Geometry: final body of the model. Coordinates: model frame, mm. A direction names the side the tool comes from. Give positions to 0.01 mm unless a question says otherwise; leave off trailing zeros. Write each loop counter-clockwise with the first axis right and the second up, starting at its lowest first coordinate (ties: lowest second). Pieces come first, ordered by that corner, then holes. Notation, with made-up numbers: M 30.25,73.5 L 59.25,73.5 A25 ccw 59.25,109.5 Z; hole C -34.5,-9.5 d11. An arc over 180 degrees is marked long. Use a Markdown table: item, result. Add a question column.
(1) Cut plane C-C (y = -119). Output: boundary loops of the cut face in (x, z), plus the area to 3 significant figures.
(2) Draft query along X for faces 1 (the flat face through (-66, -209.75, 86)), 2 (the cylindrical face through (-156.251, -140.305, 85.782)), 3 (the flat face through (163.933, -96, 86)), 4 (the cylindrical face through (185.99, -96.97, 85.78)). Return one class per face: released by +X, released by -X, zero draft, split by the parting line, or undercut.
(3) Material intervals for L1, parallel to X at y = -180, z = 83.5; L2, parallel to X at y = -142.5, z = 125; L3, parallel to Y at x = -4, z = 110.5, sorted ascending.
(4) Cut plane D-D (x = -28). Output: boundary loops of the cut face in (y, z).
(5) Pin query (flat end, axial travel): pin 1 Ø5 at (x, z) = (-42.5, 114.5) entering from -Y; pin 2 Ø10 at (x, z) = (-94.5, 102) entering from +Y; pin 3 Ø1.2 at (x, z) = (-166.5, 130) entering from -Y. Return the tip coordinate at first contact, or that it passes through.
(6) Cut plane B-B (z = 146.5). Output: boundary loops of the cut face in (x, y), plus the area to 3 significant figures.
(7) Cut plane A-A (y = -168). Output: boundary loops of the cut face in (x, z), plus the area to 3 significant figures.
(8) Reachability of faces 5 (the flat face through (-13, -199, 174)), 6 (the flat face through (120, -191, 86)), 7 (the flat face through (-163.933, -95, 86)), 8 (the flat face through (-120, -191, 86)) from +Z, -Z, +X, -X, +Y, -Y: full face, straight path, thin tool, end or side. Return the list, or none.
```python
from build123d import *

# Parameters (mm, degrees)
SKETCH_1_R          = 210
SKETCH_1_R_2        = 203
EXTRUDE_2_DEPTH     = 174
EXTRUDE_START       = -174
EXTRUDE_4_DEPTH     = 174
CUT_EXTRUDE_1_DEPTH = 654
EXTRUDE_5_DEPTH     = 174
EXTRUDE_6_DEPTH     = 174
EXTRUDE_7_DEPTH     = 174
EXTRUDE_8_DEPTH     = 174


with BuildPart() as part:
    # 草图1 → 凸台-拉伸2 (new body)
    with BuildSketch(Plane.XY):
        Circle(SKETCH_1_R)
        Circle(SKETCH_1_R_2, mode=Mode.SUBTRACT)
    extrude(amount=EXTRUDE_2_DEPTH)

    # 草图2 → 凸台-拉伸4 (add)
    with BuildSketch(Plane.XY.offset(174).offset(EXTRUDE_START)):
        with BuildLine():
            Line((-170.735431044, -102), (-173.735431044, -102))
            Line((-173.735431044, -102), (-175.513532242, -102))
            ThreePointArc((-175.513532242, -102), (-174.63092392, -103.50381834), (-173.735431044, -105))
            Line((-173.735431044, -105), (-170.735431044, -105))
            Line((-170.735431044, -105), (-170.735431044, -102))
        make_face()
        with BuildLine():
            ThreePointArc((173.735431044, -105), (174.63092392, -103.50381834), (175.513532242, -102))
            Line((175.513532242, -102), (173.735431044, -102))
            Line((173.735431044, -102), (170.735431044, -102))
            Line((170.735431044, -102), (170.735431044, -105))
            Line((170.735431044, -105), (173.735431044, -105))
        make_face()
    extrude(amount=EXTRUDE_4_DEPTH)

    # 草图3 → 切除-拉伸1 (cut)
    with BuildSketch(Plane.XY.offset(174)):
        Polygon((-170.735431044, -102), (238.333646515, -102), (254.334169784, 272.292523591), (-334.569415043, 221.85110305), (-306.830562533, -102), align=None)
    extrude(amount=-CUT_EXTRUDE_1_DEPTH, mode=Mode.SUBTRACT)

    # 草图5 → 凸台-拉伸5 (add)
    with BuildSketch(Plane.XY.offset(174).offset(EXTRUDE_START)):
        with BuildLine():
            Line((-120, -209.75), (-10.243900624, -209.75))
            ThreePointArc((-10.243900624, -209.75), (-67.755470707, -198.769203322), (-120, -172.336879396))
            Line((-120, -172.336879396), (-120, -209.75))
        make_face()
        with BuildLine():
            ThreePointArc((120, -172.336879396), (67.755470707, -198.769203322), (10.243900624, -209.75))
            Line((10.243900624, -209.75), (120, -209.75))
            Line((120, -209.75), (120, -172.336879396))
        make_face()
    extrude(amount=EXTRUDE_5_DEPTH)

    # 草图6 → 凸台-拉伸6 (add)
    with BuildSketch(Plane.XY.offset(174).offset(EXTRUDE_START)):
        with BuildLine():
            Line((-175.513532242, -102), (-166.195667814, -102))
            ThreePointArc((-166.195667814, -102), (0, -195), (166.195667814, -102))
            Line((166.195667814, -102), (175.513532242, -102))
            ThreePointArc((175.513532242, -102), (0, -203), (-175.513532242, -102))
        make_face()
    extrude(amount=EXTRUDE_6_DEPTH)

    # 草图7 → 凸台-拉伸7 (add)
    with BuildSketch(Plane.XY.offset(174).offset(EXTRUDE_START)):
        with BuildLine():
            Line((-166.933126535, -92), (-166.933126535, -95))
            Line((-166.933126535, -95), (-170.293863659, -95))
            ThreePointArc((-170.293863659, -95), (0, -195), (170.293863659, -95))
            Line((170.293863659, -95), (166.933126535, -95))
            Line((166.933126535, -95), (166.933126535, -92))
            Line((166.933126535, -92), (171.933126535, -92))
            Line((171.933126535, -92), (188.496850106, -92))
            ThreePointArc((188.496850106, -92), (0, -209.75), (-188.496850106, -92))
            Line((-188.496850106, -92), (-171.933126535, -92))
            Line((-171.933126535, -92), (-166.933126535, -92))
        make_face()
    extrude(amount=EXTRUDE_7_DEPTH)

    # 草图8 → 凸台-拉伸8 (add)
    with BuildSketch(Plane(origin=(0, 0, 0), x_dir=(-1, 0, 0), z_dir=(0, 0, -1))):
        with BuildLine():
            Line((166.933126535, -92), (163.933126535, -92))
            Line((163.933126535, -92), (163.933126535, -99))
            Line((163.933126535, -99), (168, -99))
            ThreePointArc((168, -99), (169.158755456, -97.006780447), (170.293863659, -95))
            Line((170.293863659, -95), (166.933126535, -95))
            Line((166.933126535, -95), (166.933126535, -92))
        make_face()
        with BuildLine():
            Line((-166.933126535, -95), (-170.293863659, -95))
            ThreePointArc((-170.293863659, -95), (-169.158755456, -97.006780447), (-168, -99))
            Line((-168, -99), (-163.933126535, -99))
            Line((-163.933126535, -99), (-163.933126535, -92))
            Line((-163.933126535, -92), (-166.933126535, -92))
            Line((-166.933126535, -92), (-166.933126535, -95))
        make_face()
    extrude(amount=-EXTRUDE_8_DEPTH)


solid = part.part
```
Answer list:
| question | item | result |
|---|---|---|
| 1 | outline | M -173.03,0 L -154.48,0 L -154.48,174 L -173.03,174 Z; M 154.48,0 L 173.03,0 L 173.03,174 L 154.48,174 Z |
| 1 | area | 6,460 mm² |
| 2 | face 1 | zero draft |
| 2 | face 2 | released by -X |
| 2 | face 3 | undercut |
| 2 | face 4 | released by +X |
| 3 | L1 | -120 to -75, 75 to 120 |
| 3 | L2 | -154.25 to -133.11, 133.11 to 154.25 |
| 3 | L3 | -209.96 to -194.96 |
| 4 | outline | M -209.75,0 L -192.98,0 L -192.98,174 L -209.75,174 Z |
| 5 | pin 1 | y = -209.75 |
| 5 | pin 2 | y = -167.7 |
| 5 | pin 3 | y = -128.75 |
| 6 | outline | M -188.5,-92 A209.75 ccw -183.28,-102 L -183.56,-102 A210 ccw -120,-172.34 L -120,-209.75 L -10.24,-209.75 A210 ccw 10.24,-209.75 L 120,-209.75 L 120,-172.34 A210 ccw 183.56,-102 L 183.28,-102 A209.75 ccw 188.5,-92 L 163.93,-92 L 163.93,-99 L 168,-99 A195 cw -168,-99 L -163.93,-99 L -163.93,-92 Z |
| 6 | area | 9,600 mm² |
| 7 | outline | M -126,0 L -99,0 L -99,174 L -126,174 Z; M 99,0 L 126,0 L 126,174 L 99,174 Z |
| 7 | area | 9,400 mm² |
| 8 | face 5 | +Z, +X, -X, +Y, -Y |
| 8 | face 6 | +Z, -Z, +X, -Y |
| 8 | face 7 | +Z, -Z, +Y |
| 8 | face 8 | +Z, -Z, -X, -Y |
